```python
from build123d import *

# Parameters (mm, degrees)
SKETCH2_W           = 220
SKETCH2_H           = 160
BOSS_EXTRUDE1_DEPTH = 30
SKETCH3_W           = 212
SKETCH3_H           = 152
CUT_EXTRUDE1_DEPTH  = 26
SKETCH4_W           = 300
SKETCH4_H           = 200
BOSS_EXTRUDE2_DEPTH = 5
CUT_EXTRUDE2_REACH  = 185.644
SKETCH5_R           = 2.05
SKETCH6_R           = 5
CUT_EXTRUDE3_DEPTH  = 183.14280112


with BuildPart() as part:
    # Sketch2 → Boss-Extrude1 (new body)
    with BuildSketch(Plane(origin=(0, 0, 0), x_dir=(1, 0, 0), z_dir=(0, 1, 0))):
        Rectangle(SKETCH2_W, SKETCH2_H)
    extrude(amount=BOSS_EXTRUDE1_DEPTH)

    # Sketch3 → Cut-Extrude1 (cut)
    with BuildSketch(Plane(origin=(0, 30, 0), x_dir=(1, 0, 0), z_dir=(0, 1, 0))):
        Rectangle(SKETCH3_W, SKETCH3_H)
    extrude(amount=-CUT_EXTRUDE1_DEPTH, mode=Mode.SUBTRACT)

    # Sketch4 → Boss-Extrude2 (add)
    with BuildSketch(Plane.XZ):
        Rectangle(SKETCH4_W, SKETCH4_H)
    extrude(amount=BOSS_EXTRUDE2_DEPTH)

    # Sketch5 → Cut-Extrude2 (cut, up to next)
    with BuildSketch(Plane.XZ.offset(5), mode=Mode.PRIVATE) as cut_extrude2_sk1:
        with Locations(Location((-146, 96, 0), (0, 0, 270))):
            Circle(SKETCH5_R)
    cut_extrude2_tool1 = extrude(cut_extrude2_sk1.sketch, amount=-CUT_EXTRUDE2_REACH, mode=Mode.PRIVATE) & part.part
    # Sketch5 → Cut-Extrude2 (cut, up to next)
    with BuildSketch(Plane.XZ.offset(5), mode=Mode.PRIVATE) as cut_extrude2_sk2:
        with Locations(Location((146, 96, 0), (0, 0, 90))):
            Circle(SKETCH5_R)
    cut_extrude2_tool2 = extrude(cut_extrude2_sk2.sketch, amount=-CUT_EXTRUDE2_REACH, mode=Mode.PRIVATE) & part.part
    # Sketch5 → Cut-Extrude2 (cut, up to next)
    with BuildSketch(Plane.XZ.offset(5), mode=Mode.PRIVATE) as cut_extrude2_sk3:
        with Locations(Location((146, -96, 0), (0, 0, 270))):
            Circle(SKETCH5_R)
    cut_extrude2_tool3 = extrude(cut_extrude2_sk3.sketch, amount=-CUT_EXTRUDE2_REACH, mode=Mode.PRIVATE) & part.part
    # Sketch5 → Cut-Extrude2 (cut, up to next)
    with BuildSketch(Plane.XZ.offset(5), mode=Mode.PRIVATE) as cut_extrude2_sk4:
        with Locations(Location((-146, -96, 0), (0, 0, 90))):
            Circle(SKETCH5_R)
    cut_extrude2_tool4 = extrude(cut_extrude2_sk4.sketch, amount=-CUT_EXTRUDE2_REACH, mode=Mode.PRIVATE) & part.part
    add(cut_extrude2_tool1.solids().sort_by_distance((-146, -5, 96))[0], mode=Mode.SUBTRACT)
    add(cut_extrude2_tool2.solids().sort_by_distance((146, -5, 96))[0], mode=Mode.SUBTRACT)
    add(cut_extrude2_tool3.solids().sort_by_distance((146, -5, -96))[0], mode=Mode.SUBTRACT)
    add(cut_extrude2_tool4.solids().sort_by_distance((-146, -5, -96))[0], mode=Mode.SUBTRACT)

    # Sketch6 → Cut-Extrude3 (cut, through all)
    with BuildSketch(Plane(origin=(0, 4, 0), x_dir=(1, 0, 0), z_dir=(0, 1, 0))):
        with Locations(Location((0, 0, 0), (0, 0, 270))):
            Circle(SKETCH6_R)
    extrude(amount=-CUT_EXTRUDE3_DEPTH, mode=Mode.SUBTRACT)


solid = part.part
```
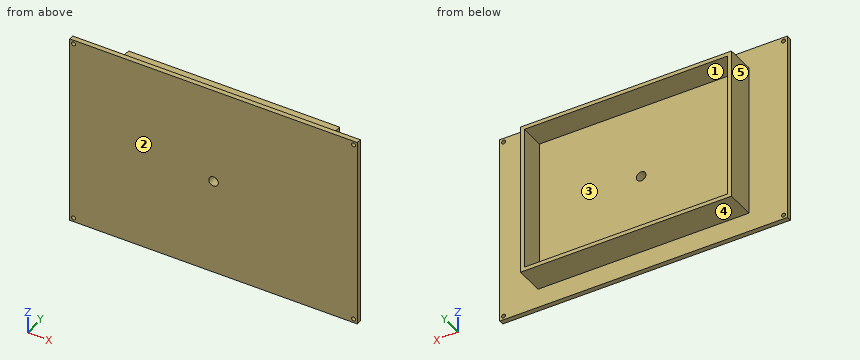
Read the model definition and answer for the solid it produces. Units are mm, in the model's axes. Face numbers are marked on the shaded views. A direction names the side the tool comes from. Give positions to 0.01 mm unless a question says otherwise; leave off trailing zeros. Order: outer loops, then holes, each group sorted by start corner. A loop starts at its lowest first (then second) coordinate and runs counter-clockwise, first axis right, second up.
(1) Find section A-A (x = 0). Give the vertices of the cut face in (y, z), plus the area to 3 significant figures.
(2) Given pin 1 (12 mm diameter, centred on x = 40.5, y = 23, fed in from +Z); pin 2 (6 mm diameter, centred on y = 10.5, z = -64, fed in from -X); pin 3 (6.5 mm diameter, centred on x = -146, z = 96, fed in from +Y); pin 4 (2.5 mm diameter, centred on x = 146, z = -96, fed in from +Y), each flat-ended and moving along its own axis, determine where each tip first touches the part or whether it passes through.
(3) Find section D-D (x = 95.5). Give the vertices of the cut face in (y, z).
(4) Find section B-B (y = 19). Give the vertices of the cut face in (x, z), plus the area to 3 significant figures.
(5) For a pull along Z with two mould halves and no side action, classify the marked faces 3, 4 and 5 as released by +Z, released by -Z, zero draft, split by the parting line, or undercut.
(6) Find section C-C (z = 9.5). Give the vertices of the cut face in (x, y), plus the area to 3 significant figures.
(7) Straight lines are drawn through the part: L1, parallel to Z at x = -146, y = -1; L2, parallel to X at y = -3, z = 96; L3, parallel to Z at x = 90, y = 18. For each, find the intervals that lie inside material, in ascending order.
(8) For the marked faces 1 and 2, determine the directions among +Z, -Z, +X, -X, +Y, -Y from which every point of the face is accessible in a straight line to the end or side of a thin tool.
Result sheet:
1. outline: (-5, -100) - (0, -100) - (0, -80) - (30, -80) - (30, -76) - (4, -76) - (4, -5) - (-5, -5) - close; (-5, 5) - (4, 5) - (4, 76) - (30, 76) - (30, 80) - (0, 80) - (0, 100) - (-5, 100) - close
1. area: 1,760 mm2
2. pin 1: stops at z = 80
2. pin 2: stops at x = -110
2. pin 3: stops at y = 0
2. pin 4: passes through
3. outline: (-5, -100) - (0, -100) - (0, -80) - (30, -80) - (30, -76) - (4, -76) - (4, 76) - (30, 76) - (30, 80) - (0, 80) - (0, 100) - (-5, 100) - close
4. outline: (-110, -80) - (110, -80) - (110, 80) - (-110, 80) - close; hole (-106, -76) - (106, -76) - (106, 76) - (-106, 76) - close
4. area: 2,980 mm2
5. face 3: undercut
5. face 4: released by -Z
5. face 5: zero draft
6. outline: (-150, -5) - (150, -5) - (150, 0) - (110, 0) - (110, 30) - (106, 30) - (106, 4) - (-106, 4) - (-106, 30) - (-110, 30) - (-110, 0) - (-150, 0) - close
6. area: 2,590 mm2
7. L1: z = -100 to -98.05, -93.95 to 93.95, 98.05 to 100
7. L2: x = -150 to -148.05, -143.95 to 143.95, 148.05 to 150
7. L3: z = -80 to -76, 76 to 80
8. face 1: +Y
8. face 2: +Z, -Z, +X, -X, -Y
